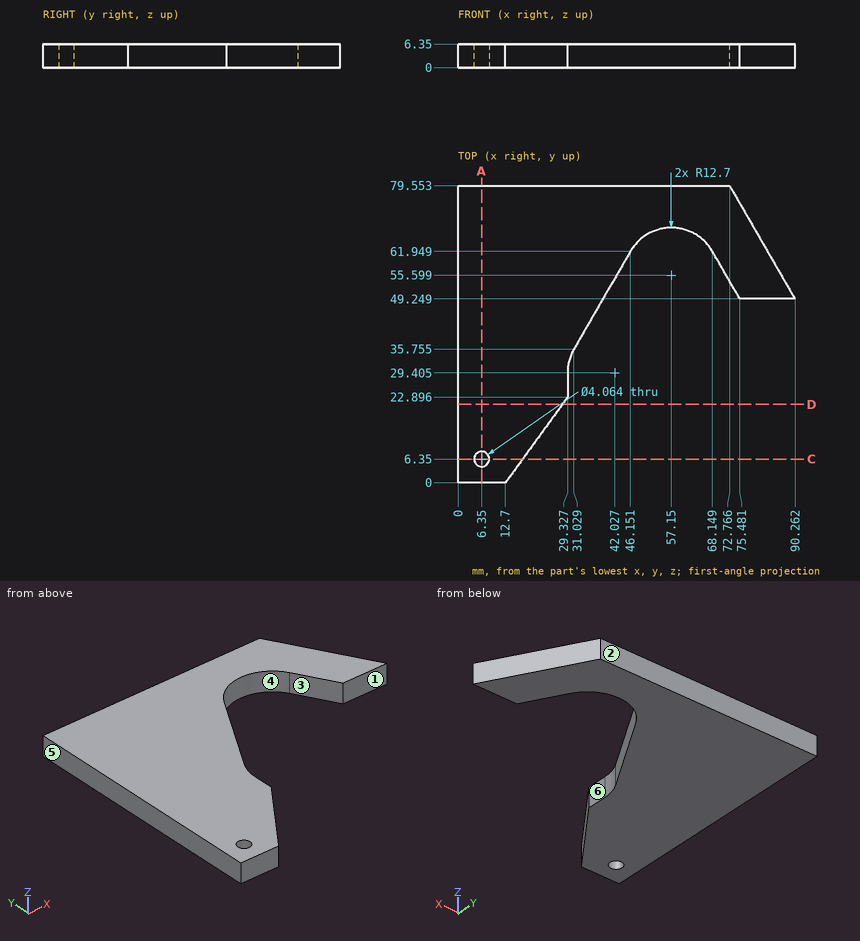
Drawing for the job (mm, zero at the part's lowest x, y, z). A direction names the side the tool comes from. Round coordinates to 2 decimals unless told otherwise and drop trailing zeros. Order: outer loops, then holes, each group sorted by start corner. A loop starts at its lowest first (then second) coordinate and runs counter-clockwise, first axis right, second up. Notation, with made-up numbers: (82.5, 29) -> (120.5, 29) arc R28 ccw to (120.5, 55) -> close; hole circle Ø1 at (76, -1.5). An arc over 180 degrees is marked (long way). Write item = value, one per line. Start each with the question number.
(1) Pin check, flat tips, straight feed: P1, Ø1.5, axis at y = 65, z = 1, coming from the +X side; P2, Ø1, axis at y = 53, z = 4, coming from the +X side (1 decimal); P3, Ø3, axis at y = 24.5, z = 2.5, coming from the +X side. Stop position of each tip, or through.
(2) Cut at D-D, the plane y = 21. List the corners of the cut face in (x, z).
(3) Cut at C-C, the plane y = 6.35. List the corners of the cut face in (x, z).
(4) Which spindle directions (+Z, -Z, +X, -X, +Y, -Y) get a long thin tool onto all of the face, cutting with end or side? Do the marked faces 1, 2 and 3. Say none if no direction does.
(5) Probe line 1 (Y direction, x = 6.35, z = 4.75); line 2 (X direction, y = 29, z = 4.5); line 3 (Y direction, x = 59, z = 2.25). List the from-to ranges inside material, lowest first. Write a range as [from, to].
(6) Cut at A-A, the plane x = 6.35. List the corners of the cut face in (y, z).
(7) Pull direction X, two halves, no side cores. Call the marked faces 4, 5 and 6: released by +X, released by -X, zero draft, split by the parting line, or undercut.
Model answer:
q1.P1 = 81.6
q1.P2 = 88.4
q1.P3 = 29.33
q2.outline = (0, 0) -> (27.95, 0) -> (27.95, 6.35) -> (0, 6.35) -> close
q3.outline = (0, 0) -> (4.32, 0) -> (4.32, 6.35) -> (0, 6.35) -> close; (8.38, 0) -> (17.31, 0) -> (17.31, 6.35) -> (8.38, 6.35) -> close
q4.face_1 = +Z, -Z, +X, -Y
q4.face_2 = +Z, -Z, +X, -X, +Y
q4.face_3 = +Z, -Z, -Y
q5.line_1 = [0, 4.32], [8.38, 79.55]
q5.line_2 = [0, 29.33]
q5.line_3 = [68.16, 79.55]
q6.outline = (0, 0) -> (4.32, 0) -> (4.32, 6.35) -> (0, 6.35) -> close; (8.38, 0) -> (79.55, 0) -> (79.55, 6.35) -> (8.38, 6.35) -> close
q7.face_4 = undercut
q7.face_5 = released by -X
q7.face_6 = released by +X
